Source: CAD feature listing. Evaluate the final solid. Frame: model axes, mm. A direction names the side the tool comes from. Give positions to 0.01 mm unless a question says otherwise; leave off trailing zeros. Loops run counter-clockwise (first coordinate to the right, second up) from the corner with the lowest first, then second, coordinate; pieces in that order, holes last. Notation, with made-up numbers: M -34.5,48 L -1.5,48 A26 cw -1.5,65 Z; hole C -10,-29.75 d8. An arc over 180 degrees is marked long. Put each result on its own line as item: value.
from build123d import *

# Parameters (mm, degrees)
F1_DEPTH = 34
F2_W     = 6.5
F2_H     = 30
F3_DEPTH = 8
F4_R     = 3.5
F5_DEPTH = 6
F6_W     = 42
F6_H     = 10
F6_H_2   = 6
F7_DEPTH = 30
F8_SIZE  = 3
F9_SIZE  = 2
F10_SIZE = 1


with BuildPart() as f1:
    # F0 (on Front) → F1 (new body)
    with BuildSketch(Plane.XZ):
        Polygon((-20, 8), (-25, 8), (-25, -8), (25, -8), (25, 38), (17, 38), (17, 8), align=None)
    extrude(amount=F1_DEPTH)

    # F2 (on face) → F3 (cut, through all)
    with BuildSketch(Plane.YZ.offset(25)):
        with Locations((-17, 23)):
            Rectangle(F2_W, F2_H)
    extrude(amount=-F3_DEPTH, mode=Mode.SUBTRACT)

    # F4 (on face) → F5 (cut)
    with BuildSketch(Plane(origin=(-25, 0, 0), x_dir=(0, -1, 0), z_dir=(-1, 0, 0))):
        with Locations((17, 0)):
            Circle(F4_R)
    extrude(amount=-F5_DEPTH, mode=Mode.SUBTRACT)

    # F6 (on face) → F7 (join, through all)
    with BuildSketch(Plane.XY.offset(8)):
        with Locations((-4, -29)):
            Rectangle(F6_W, F6_H)
        with Locations((-4, -3)):
            Rectangle(F6_W, F6_H_2)
    extrude(amount=F7_DEPTH)

    # F8
    f8_edges = [f1.edges().sort_by_distance(p)[0] for p in [
        (-4, -24, 38),
        (-4, -6, 38),
    ]]
    chamfer(f8_edges, length=F8_SIZE)

    # F9
    f9_edges = [f1.edges().sort_by_distance(p)[0] for p in [
        (25, -34, 15),
        (25, 0, 15),
        (-25, -34, 15),
        (-25, 0, 15),
    ]]
    chamfer(f9_edges, length=F9_SIZE)

    # F10
    f10_edges = [f1.edges().sort_by_distance(p)[0] for p in [
        (17, -13.75, 23),
        (17, -20.25, 23),
        (25, -13.75, 23),
        (25, -20.25, 23),
    ]]
    chamfer(f10_edges, length=F10_SIZE)


solid = f1.part
1. Section query A-A (z = 9). Output: boundary loops of the cut face in (x, y), plus the area to 3 significant figures.
Found:
outline: M -25,-32 L -23,-34 L 23,-34 L 25,-32 L 25,-21.25 L 24,-20.25 L 18,-20.25 L 17,-21.25 L 17,-24 L -25,-24 Z; M -25,-6 L 17,-6 L 17,-12.75 L 18,-13.75 L 24,-13.75 L 25,-12.75 L 25,-2 L 23,0 L -23,0 L -25,-2 Z
area: 882 mm^2
2. Section query B-B (y = -17). Output: boundary loops of the cut face in (x, z), plus the area to 3 significant figures.
Found:
outline: M -25,-8 L 25,-8 L 25,8 L -25,8 L -25,3.5 L -19,3.5 L -19,-3.5 L -25,-3.5 Z
area: 758 mm^2
3. Access query for faces 4 (the flat face through (-25, -17, 4)), 5 (the flat face through (-4, -24, 21)), 6 (the flat face through (-19, -17, 0)), 7 (the flat face through (21, -13.75, 23)), 8 (the flat face through (7.3, -2.8, 38)). Directions: +Z, -Z, +X, -X, +Y, -Y. A direction counts if a zero-diameter tool reaches every point of the face in a straight line with its end or side. Return the directions, or none.
Found:
face 4: +Z, -Z, -X, +Y, -Y
face 5: +Z, -X
face 6: -X
face 7: +Z, +X, -X
face 8: +Z, +X, -X, +Y, -Y
4. Draft query along Z for faces 1 (the cylindrical face through (-22.04, -20.34, 1.05)), 2 (the flat face through (24, -1, 15)), 3 (the flat face through (0, -17, -8)). Return one class per face: pulls with the +Z half, pulls with the -Z half, needs draft (parallel to the pull), parting line crosses it, or undercut.
Found:
face 1: undercut
face 2: needs draft
face 3: pulls with the -Z half
5. Section query D-D (z = 0). Output: boundary loops of the cut face in (x, y), plus the area to 3 significant figures.
Found:
outline: M -25,-32 L -23,-34 L 23,-34 L 25,-32 L 25,-2 L 23,0 L -23,0 L -25,-2 L -25,-13.5 L -19,-13.5 L -19,-20.5 L -25,-20.5 Z
area: 1,650 mm^2
6. Material intervals for line 1 (Z direction, x = -23.1, y = -17); line 2 (Y direction, x = -1, z = 29); line 3 (Z direction, x = 16.5, y = -16), sorted ascending. Write a range as from..to.
Found:
line 1: -8..-3.5, 3.5..8
line 2: -34..-24, -6..0
line 3: -8..8
7. Contact query for a flat-ended pin moving along its axis: P1, Ø3, axis at y = -8.5, z = 26, coming from the -X side. Output: stop coordinate, or through.
Found:
P1: x = 17
8. Section query C-C (x = 20). Output: boundary loops of the cut face in (y, z).
Found:
outline: M -34,-8 L 0,-8 L 0,38 L -13.75,38 L -13.75,8 L -20.25,8 L -20.25,38 L -34,38 Z
